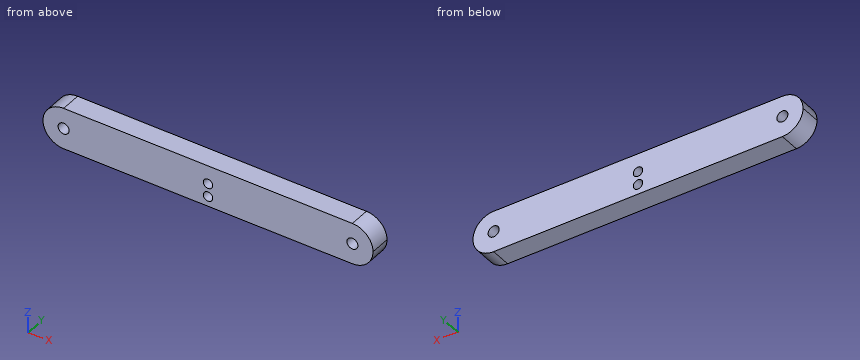
```python
from build123d import *

# Parameters (mm, degrees)
SKETCH1_R               = 1.7
BOSS_EXTRUDE1_DEPTH     = 6.35
FILLET1_R               = 6.35
CUT_EXTRUDE1_DEPTH      = 52.587643869
CUT_EXTRUDE1_DEPTH_BACK = 52.587643869
SKETCH3_R               = 1.45


with BuildPart() as part:
    # Sketch1 → Boss-Extrude1 (new body)
    with BuildSketch(Plane(origin=(0, 0, 0), x_dir=(1, 0, 0), z_dir=(0, 1, 0))):
        Polygon((-50.8, 6.35), (-50.8, -6.35), (-6.35, -6.35), (6.35, -6.35), (50.8, -6.35), (50.8, 6.35), (6.35, 6.35), (-6.35, 6.35), align=None)
        with Locations(Location((-44.45, 0, 0), (0, 0, 270))):
            Circle(SKETCH1_R, mode=Mode.SUBTRACT)
        with Locations(Location((44.45, 0, 0), (0, 0, 270))):
            Circle(SKETCH1_R, mode=Mode.SUBTRACT)
    extrude(amount=BOSS_EXTRUDE1_DEPTH)

    # Fillet1
    fillet1_edges = [part.edges().sort_by_distance(p)[0] for p in [
        (50.8, 3.175, -6.35),
        (-50.8, 3.175, -6.35),
        (-50.8, 3.175, 6.35),
        (50.8, 3.175, 6.35),
    ]]
    fillet(fillet1_edges, radius=FILLET1_R - 0.0001)  # a hair under: the kernel refuses the full size

    # Sketch3 → Cut-Extrude1 (cut, two sides: drawn at the far end of the back side and taken through both)
    with BuildSketch(Plane(origin=(0, 6.35, 0), x_dir=(1, 0, 0), z_dir=(0, 1, 0)).offset(-CUT_EXTRUDE1_DEPTH_BACK)):
        with Locations(Location((0, -0.704506674, 0), (0, 0, 270))):
            Circle(SKETCH3_R)
        with Locations(Location((0, 3.295493326, 0), (0, 0, 270))):
            Circle(SKETCH3_R)
    extrude(amount=CUT_EXTRUDE1_DEPTH + CUT_EXTRUDE1_DEPTH_BACK, mode=Mode.SUBTRACT)


solid = part.part
```
Source: CAD feature listing. Evaluate the final solid. Frame: model axes, mm. Coordinates: 2 decimals unless noted, no trailing zeros. Order: outer loops, then holes, each group sorted by start corner. A loop starts at its lowest first (then second) coordinate and runs counter-clockwise, first axis right, second up. Notation, with made-up numbers: (50, 2.25) - (80, 2.25) arc R17 ccw to (80, 19.25) - close; hole circle Ø3 at (8, 32.25). An arc over 180 degrees is marked (long way). One line per item, written item: value.
1) Contact query for flat-ended pins moving along their axis: pin 1 (2 mm diameter, centred on y = 3.5, z = 2, fed in from +X); pin 2 (2.5 mm diameter, centred on x = 0, z = 0.7, fed in from -Y). Output: stop coordinate, or through.
Computed values:
pin 1: stops at x = 50.72
pin 2: passes through
2) Ray query, line 1 (Z direction, x = 0, y = 4.75); line 2 (X direction, y = 4.5, z = 0); line 3 (X direction, y = 4.75, z = 1.25). Return the intervals inside material, ascending. Write a range as [from, to].
Computed values:
line 1: z = [-6.35, -4.75], [-1.85, -0.75], [2.15, 6.35]
line 2: x = [-50.8, -46.15], [-42.75, -1.27], [1.27, 42.75], [46.15, 50.8]
line 3: x = [-50.68, -45.6], [-43.3, -1.34], [1.34, 43.3], [45.6, 50.68]
3) Cut plane C-C on z = 4.25. Output: boundary loops of the cut face in (x, y), plus the area to 3 significant figures.
Computed values:
outline: (-49.17, 0) - (49.17, 0) - (49.17, 6.35) - (-49.17, 6.35) - close
area: 624 mm^2
4) Cut plane A-A on y = 1.5. State how many separate pieces and enclosed holes the cut face has, plus the area to 3 significant figures.
Computed values:
separate pieces: 1
enclosed holes: 4
area: 1,220 mm^2
5) Cut plane B-B on x = 0. Output: boundary loops of the cut face in (y, z), plus the area to 3 significant figures.
Computed values:
outline: (0, -6.35) - (6.35, -6.35) - (6.35, -4.75) - (0, -4.75) - close; (0, -1.85) - (6.35, -1.85) - (6.35, -0.75) - (0, -0.75) - close; (0, 2.15) - (6.35, 2.15) - (6.35, 6.35) - (0, 6.35) - close
area: 43.8 mm^2
